from build123d import *

# Parameters (mm, degrees)
SKETCH1_W                  = 127
SKETCH1_H                  = 8.636
BOSS_EXTRUDE1_DEPTH        = 101.6
SKETCH3_W                  = 8.7376
SKETCH3_H                  = 118.364
BOSS_EXTRUDE2_DEPTH        = 101.6
F_1_2_0_5000_DOWEL_HOLE2_D = 12.7
F_3_8_0_3750_DOWEL_HOLE3_D = 9.525


with BuildPart() as part:
    # Sketch1 → Boss-Extrude1 (new body)
    with BuildSketch(Plane.XY):
        Rectangle(SKETCH1_W, SKETCH1_H)
    extrude(amount=BOSS_EXTRUDE1_DEPTH)

    # Sketch3 → Boss-Extrude2 (add, through all)
    with BuildSketch(Plane.XY.offset(101.6)):
        with Locations((59.1312, 63.5)):
            Rectangle(SKETCH3_W, SKETCH3_H)
    extrude(amount=-BOSS_EXTRUDE2_DEPTH)

    # 1/2 (0.5000) Dowel Hole2 (through all)
    with Locations(Plane(origin=(16.6624, 4.318, 50.8), x_dir=(0, 0, 1), z_dir=(0, 1, 0))):
        with Locations((0, 0)):
            Hole(F_1_2_0_5000_DOWEL_HOLE2_D / 2)

    # 3/8 (0.3750) Dowel Hole3 (through all)
    with Locations(Plane(origin=(54.7624, 45.593, 52.765386082), x_dir=(0, 0, -1), z_dir=(-1, 0, 0))):
        with Locations((0, 0)):
            Hole(F_3_8_0_3750_DOWEL_HOLE3_D / 2)


solid = part.part
The listing builds one solid part. Answer for the finished solid, in the listing's coordinates (mm). A direction names the side the tool comes from. Give positions to 0.01 mm unless a question says otherwise; leave off trailing zeros. Write each loop counter-clockwise with the first axis right and the second up, starting at its lowest first coordinate (ties: lowest second). Pieces come first, ordered by that corner, then holes. Notation, with made-up numbers: (-1.5, 46.25) -> (14.5, 46.25) arc R23 cw to (14.5, 75.25) -> close; hole circle Ø3 at (15.5, 81). An arc over 180 degrees is marked (long way). Use a Markdown table: item, result.
(1) Section A-A, the plane z = 54 is taken. Determine the outline of the cut face in (x, y).
Return value:
| item | result |
|---|---|
| outline | (-63.5, -4.32) -> (11.18, -4.32) -> (11.18, 4.32) -> (-63.5, 4.32) -> close; (22.15, -4.32) -> (63.5, -4.32) -> (63.5, 40.99) -> (54.76, 40.99) -> (54.76, 4.32) -> (22.15, 4.32) -> close; (54.76, 50.19) -> (63.5, 50.19) -> (63.5, 122.68) -> (54.76, 122.68) -> close |
(2) Section C-C, the plane z = 22.5 is taken. Determine the outline of the cut face in (x, y), then the cut area to 3 significant figures.
Return value:
| item | result |
|---|---|
| outline | (-63.5, -4.32) -> (63.5, -4.32) -> (63.5, 122.68) -> (54.76, 122.68) -> (54.76, 4.32) -> (-63.5, 4.32) -> close |
| area | 2,130 mm2 |
(3) Find the intervals of material crossed by probe 1 along X at (y, z) = (84, 10); probe 2 along Y at (x, z) = (-3, 15); probe 3 along X at (y, z) = (2, 50), in increasing order. Write a range as from..to.
Return value:
| item | result |
|---|---|
| probe 1 | 54.76..63.5 |
| probe 2 | -4.32..4.32 |
| probe 3 | -63.5..10.36, 22.96..63.5 |
(4) Section B-B, the plane x = 21 is taken. Determine the outline of the cut face in (y, z).
Return value:
| item | result |
|---|---|
| outline | (-4.32, 0) -> (4.32, 0) -> (4.32, 46.16) -> (-4.32, 46.16) -> close; (-4.32, 55.44) -> (4.32, 55.44) -> (4.32, 101.6) -> (-4.32, 101.6) -> close |
(5) Flat-ended cylindrical pins translate along their axes: P1, Ø7.5, axis at x = 16.66, z = 50.8, coming from the +Y side; P2, Ø8, axis at y = 58, z = 49.5, coming from the -X side; P3, Ø1, axis at x = -6, z = 22.5, coming from the +Y side. Find the tip coordinate at first contact, or state that the pin passes through.
Return value:
| item | result |
|---|---|
| P1 | through |
| P2 | x = 54.76 |
| P3 | y = 4.32 |
(6) Section D-D, the plane y = 111.5 is taken. Determine the outline of the cut face in (x, z).
Return value:
| item | result |
|---|---|
| outline | (54.76, 0) -> (63.5, 0) -> (63.5, 101.6) -> (54.76, 101.6) -> close |
(7) For faces 1 (the flat face through (54.762, 63, 52)), 2 (the flat face through (63.5, 58, 52)), determine the directions among +Z, -Z, +X, -X, +Y, -Y from which every point of the face is accessible in a straight line to the end or side of a thin tool.
Return value:
| item | result |
|---|---|
| face 1 | +Z, -Z, -X, +Y |
| face 2 | +Z, -Z, +X, +Y, -Y |
(8) Determine the mould class of faces 3 (the flat face through (-5, 4.318, 50)), 4 (the flat face through (28, 3, 0)), 5 (the cylindrical face through (18.57, -0.06, 44.743)) for opening direction Z: released by +Z, released by -Z, zero draft, split by the parting line, or undercut.
Return value:
| item | result |
|---|---|
| face 3 | zero draft |
| face 4 | released by -Z |
| face 5 | undercut |
